```python
from build123d import *

# Parameters (mm, degrees)
F0_R     = 12
F0_R_2   = 2
F1_DEPTH = 15
F2_SIZE  = 1
F3_R     = 5
F4_DEPTH = 3
F5_R     = 4
F6_DEPTH = 3


with BuildPart() as f1:
    # F0 (on Top) → F1 (new body)
    with BuildSketch(Plane.XY):
        Circle(F0_R)
        Circle(F0_R_2, mode=Mode.SUBTRACT)
    extrude(amount=-F1_DEPTH)

    # F2
    f2_edges = [f1.edges().sort_by_distance(p)[0] for p in [
        (-12, 0, -15),
        (-12, 0, 0),
    ]]
    chamfer(f2_edges, length=F2_SIZE)

    # F3 (on face) → F4 (cut)
    with BuildSketch(Plane.XY):
        Circle(F3_R)
    extrude(amount=-F4_DEPTH, mode=Mode.SUBTRACT)

    # F5 (on face) → F6 (cut)
    with BuildSketch(Plane(origin=(0, 0, -15), x_dir=(1, 0, 0), z_dir=(0, 0, -1))):
        Circle(F5_R)
    extrude(amount=-F6_DEPTH, mode=Mode.SUBTRACT)


solid = f1.part
```
Could you check a few things on this model? Use its own coordinates, in mm. A direction names the side the tool comes from. Coordinates: 2 decimals unless noted, no trailing zeros. Write each loop counter-clockwise with the first axis right and the second up, starting at its lowest first coordinate (ties: lowest second). Pieces come first, ordered by that corner, then holes. Notation, with made-up numbers: (52.5, 29.5) - (109.5, 29.5) arc R17 ccw to (109.5, 44.5) - close; hole circle Ø6 at (-31.75, 62). An arc over 180 degrees is marked (long way). Use a Markdown table: item, result.
Q1. Please list where these lines run through material, in increasing order: L1, parallel to Y at x = 0, z = -13.5; L2, parallel to Y at x = 0, z = -8.75; L3, parallel to Y at x = 10.5, z = -6.5.
Geometry check:
| item | result |
|---|---|
| L1 | y = -12 to -4, 4 to 12 |
| L2 | y = -12 to -2, 2 to 12 |
| L3 | y = -5.81 to 5.81 |
Q2. Imagine slicing it at A-A (x = 0). List the corners of the cut face in (y, z) for me, and give its area (3 significant figures).
Geometry check:
| item | result |
|---|---|
| outline | (-12, -14) - (-11, -15) - (-4, -15) - (-4, -12) - (-2, -12) - (-2, -3) - (-5, -3) - (-5, 0) - (-11, 0) - (-12, -1) - close; (2, -12) - (4, -12) - (4, -15) - (11, -15) - (12, -14) - (12, -1) - (11, 0) - (5, 0) - (5, -3) - (2, -3) - close |
| area | 268 mm2 |
Q3. I'm going to push flat-ended pins straight in: pin 1 Ø5 at (x, y) = (0, 0) entering from -Z; pin 2 Ø8 at (x, y) = (0, 0) entering from +Z; pin 3 Ø2 at (x, z) = (-6, -8) entering from -Y. Where does each tip first touch, or does it pass through?
Geometry check:
| item | result |
|---|---|
| pin 1 | stops at z = -12 |
| pin 2 | stops at z = -3 |
| pin 3 | stops at y = -10.91 |
Q4. Which directions (+Z, -Z, +X, -X, +Y, -Y) give clear straight access to the entire face, cutting with the end or side of a thin tool? Please do faces 4 (the flat face through (-2, 1, -12)), 5 (the flat face through (2, -5, 0)), 6 (the cylindrical face through (-1.08, -4.88, -1.48)).
Geometry check:
| item | result |
|---|---|
| face 4 | -Z |
| face 5 | +Z, +X, -X, +Y, -Y |
| face 6 | +Z |
Q5. Thinking about a two-plate mould opening in Y: for faces 1 (the cylindrical face through (0, -2, -7)), 2 (the flat face through (0, -5, -15)), 3 (the cylindrical face through (-11.99, 0.53, -7.41)), which applies, +Y half, -Y half, draft (parallel to the pull), parting line (faces both ways), or undercut?
Geometry check:
| item | result |
|---|---|
| face 1 | undercut |
| face 2 | draft |
| face 3 | parting line |
Q6. Imagine slicing it at C-C (z = -11.5). List the corners of the cut face in (x, y) for me.
Geometry check:
| item | result |
|---|---|
| outline | circle Ø24 at (0, 0); hole circle Ø4 at (0, 0) |
